Could you check a few things on this drawing? It's one solid part, dimensions in mm from its lowest x, y, z. Give positions to 0.01 mm unless a question says otherwise; leave off trailing zeros. Loops run counter-clockwise (first coordinate to the right, second up) from the corner with the lowest first, then second, coordinate; pieces in that order, holes last. Notation, with made-up numbers: (-23, 58.25) - (-9, 58.25) arc R29 ccw to (-9, 81.25) - close; hole circle Ø3 at (1, -24.5). An arc over 180 degrees is marked (long way). Answer as a JSON object with one key per item and string values.
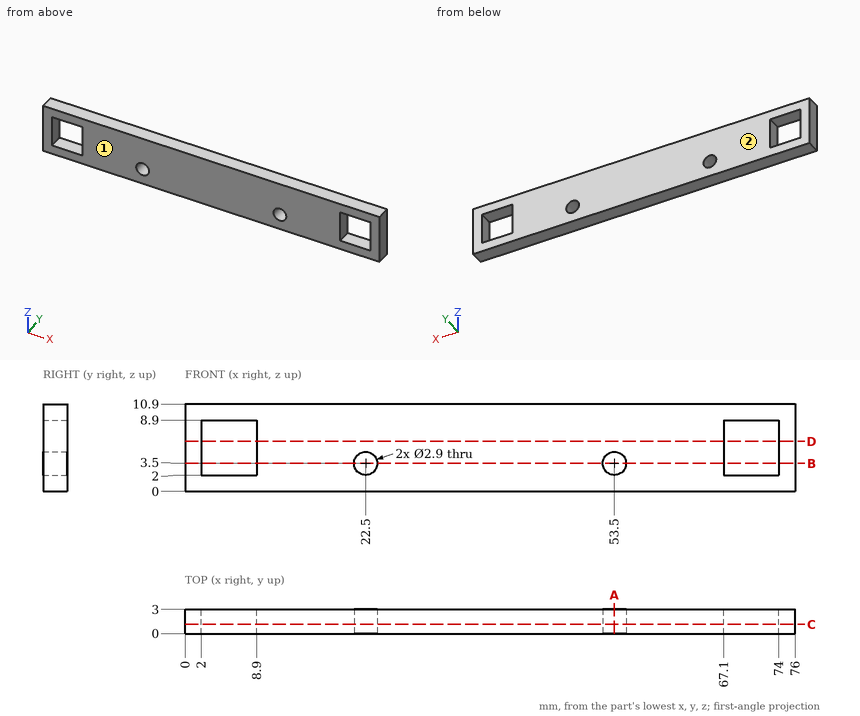
1) Imagine slicing it at B-B on z = 3.5. Write out the boundary of the cut face in (x, y).
Check sheet entries:
{"outline": "(0, 0) - (2, 0) - (2, 3) - (0, 3) - close; (8.9, 0) - (21.05, 0) - (21.05, 3) - (8.9, 3) - close; (23.95, 0) - (52.05, 0) - (52.05, 3) - (23.95, 3) - close; (54.95, 0) - (67.1, 0) - (67.1, 3) - (54.95, 3) - close; (74, 0) - (76, 0) - (76, 3) - (74, 3) - close"}
2) Imagine slicing it at C-C on y = 1.15. Write out the boundary of the cut face in (x, z), and give its area (3 significant figures).
Check sheet entries:
{"outline": "(0, 0) - (76, 0) - (76, 10.9) - (0, 10.9) - close; hole (2, 2) - (8.9, 2) - (8.9, 8.9) - (2, 8.9) - close; hole circle Ø2.9 at (22.5, 3.5); hole circle Ø2.9 at (53.5, 3.5); hole (67.1, 2) - (74, 2) - (74, 8.9) - (67.1, 8.9) - close", "area": "720 mm2"}
3) Imagine slicing it at A-A on x = 53.5. Write out the boundary of the cut face in (y, z), and give its area (3 significant figures).
Check sheet entries:
{"outline": "(0, 0) - (3, 0) - (3, 2.05) - (0, 2.05) - close; (0, 4.95) - (3, 4.95) - (3, 10.9) - (0, 10.9) - close", "area": "24.0 mm2"}
4) Imagine slicing it at D-D on z = 6.25. Write out the boundary of the cut face in (x, y), and give its area (3 significant figures).
Check sheet entries:
{"outline": "(0, 0) - (2, 0) - (2, 3) - (0, 3) - close; (8.9, 0) - (67.1, 0) - (67.1, 3) - (8.9, 3) - close; (74, 0) - (76, 0) - (76, 3) - (74, 3) - close", "area": "187 mm2"}
5) If we mould it in two halves opening along Y, with no side actions, what happens to the marked faces 1 and 2? For each: released by +Y, released by -Y, zero draft, split by the parting line, or undercut.
Check sheet entries:
{"face 1": "released by -Y", "face 2": "released by +Y"}
6) I need wall thicknesses on L1, parallel to X at y = 2.55, z = 8.5; L2, parallel to X at y = 0.6, z = 3.5; L3, parallel to Z at x = 53.5, y = 1.25. Which ranges of each line are inside material? Lowest first, please.
Check sheet entries:
{"L1": "0 to 2, 8.9 to 67.1, 74 to 76", "L2": "0 to 2, 8.9 to 21.05, 23.95 to 52.05, 54.95 to 67.1, 74 to 76", "L3": "0 to 2.05, 4.95 to 10.9"}
7) I'm going to push a flat-ended pin straight in: P1, Ø1.7, axis at x = 53.5, z = 3.5, coming from the +Y side. Where does the tip first touch, or does it pass through?
Check sheet entries:
{"P1": "through"}
